from build123d import *

# Parameters (mm, degrees)
SKETCH1_R                = 2.75
BOSS_EXTRUDE1_DEPTH      = 12
BOSS_EXTRUDE2_DEPTH      = 30
BOSS_EXTRUDE2_DEPTH_BACK = 10
CHAMFER1_SIZE            = 17.501152045
CHAMFER1_SIZE_2          = 15
SKETCH4_R                = 2
CUT_EXTRUDE1_DEPTH       = 30
CHAMFER2_SIZE            = 1.5
CUT_EXTRUDE2_DEPTH       = 30
CUT_EXTRUDE2_DEPTH_BACK  = 4
SKETCH5_R                = 5.5
CHAMFER3_SIZE            = 3
BOSS_EXTRUDE3_DEPTH      = 10


with BuildPart() as part:
    # Sketch1 → Boss-Extrude1 (new body)
    with BuildSketch(Plane.XY):
        with BuildLine():
            Line((0, 55), (-15, 55))
            Line((-15, 55), (-10.865898, 24.40520649))
            Line((-10.865898, 24.40520649), (-9.354942791, 21.011545526))
            ThreePointArc((-9.354942791, 21.011545526), (-9.852249787, 20.783002048), (-10.343977944, 20.542690191))
            Line((-10.343977944, 20.542690191), (-7.432453853, -1.004305596))
            ThreePointArc((-7.432453853, -1.004305596), (-4.935468976, -5.647224627), (0, -7.5))
            Line((0, -7.5), (0, -2.75))
            ThreePointArc((0, -2.75), (-2.75, 0), (0, 2.75))
            Line((0, 2.75), (0, 55))
        make_face()
        with Locations((-6.077686218, 34.468271355)):
            Circle(SKETCH1_R, mode=Mode.SUBTRACT)
    extrude(amount=BOSS_EXTRUDE1_DEPTH)

    # Sketch3 → Boss-Extrude2 (add, two sides: drawn at the far end of the back side and taken through both)
    with BuildSketch(Plane(origin=(0, 55, 0), x_dir=(1, 0, 0), z_dir=(0, 1, 0)).offset(-BOSS_EXTRUDE2_DEPTH_BACK)):
        Polygon((0, -17), (-19.25, -17), (-19.25, 10), (-11.25, 10), (-11.25, -12), (0, -12), align=None)
    extrude(amount=BOSS_EXTRUDE2_DEPTH + BOSS_EXTRUDE2_DEPTH_BACK)

    # Chamfer1
    # the kernel refuses this chamfer: 17.501152045, 15 mm, written as the material it adds along each edge
    with BuildSketch(Plane(origin=(-13.648756365, 45, 12), x_dir=(0.1571469904838525, -0.9875752241636421, 0), z_dir=(0, 0, -1))) as chamfer1_piece_1_section:
        Polygon((CHAMFER1_SIZE * 0.999724117502, CHAMFER1_SIZE * 0.0234880574124), (-CHAMFER1_SIZE_2 * 0.157146990484, CHAMFER1_SIZE_2 * 0.987575224164), (0, 0), align=None)
    chamfer1_piece_1 = extrude(amount=12, mode=Mode.PRIVATE)
    chamfer1_piece_1 = split(chamfer1_piece_1, bisect_by=Plane(origin=(-19.25, 37.743808278, 6), z_dir=(1, 0, 0)), keep=Keep.TOP, mode=Mode.PRIVATE)
    add(chamfer1_piece_1)
    # the kernel refuses this chamfer: 17.501152045, 15 mm, written as the material it adds along each edge
    with BuildSketch(Plane(origin=(0, 45, 12), x_dir=(0, 0.02749587661058632, 0.9996219169112968), z_dir=(-1, 0, 0))) as chamfer1_2_piece_1_section:
        Polygon((CHAMFER1_SIZE_2 * 0.999621916911, -CHAMFER1_SIZE_2 * 0.0274958766106), (-CHAMFER1_SIZE_2 * 0.0274958766106, -CHAMFER1_SIZE_2 * 0.999621916911), (0, 0), align=None)
    chamfer1_2_piece_1 = extrude(amount=19.25, mode=Mode.PRIVATE)
    chamfer1_2_piece_1 = chamfer1_2_piece_1 - Plane(origin=(-6.077686218, 34.468271355, 14.181154437), x_dir=(1, 0, 0), z_dir=(0, 0, -1)) * Cylinder(2.75, 99, mode=Mode.PRIVATE)
    chamfer1_2_piece_1 = split(chamfer1_2_piece_1, bisect_by=Plane(origin=(-16.223862411, 32.575106046, 14.181154437), z_dir=(0.7071067811865486, 0.7071067811865466, 0)), keep=Keep.TOP, mode=Mode.PRIVATE)
    chamfer1_2_piece_1 = split(chamfer1_2_piece_1, bisect_by=Plane(origin=(-9.68028065, 39.118687807, 17), z_dir=(0, 0, -1)), keep=Keep.TOP, mode=Mode.PRIVATE)
    add(chamfer1_2_piece_1)

    # Sketch4 → Cut-Extrude1 (cut)
    with BuildSketch(Plane.ZY.offset(19.25)):
        with Locations((1, 70)):
            Circle(SKETCH4_R)
    extrude(amount=-CUT_EXTRUDE1_DEPTH, mode=Mode.SUBTRACT)

    # Chamfer2
    chamfer2_edges = [part.edges().sort_by_distance(p)[0] for p in [
        (-19.25, 70, -1),
    ]]
    chamfer(chamfer2_edges, length=CHAMFER2_SIZE)

    # Sketch5 → Cut-Extrude2 (cut, two sides: drawn at the far end of the back side and taken through both)
    with BuildSketch(Plane.XY.offset(12).offset(-CUT_EXTRUDE2_DEPTH_BACK)):
        Circle(SKETCH5_R)
        with Locations(Location((-6.077686218, 34.468271355, 0), (0, 0, 180))):
            Circle(SKETCH5_R)
    extrude(amount=CUT_EXTRUDE2_DEPTH + CUT_EXTRUDE2_DEPTH_BACK, mode=Mode.SUBTRACT)

    # Chamfer3
    # the kernel refuses this chamfer: 3 mm, written as the material it takes off along each edge
    with BuildSketch(Plane(origin=(0, 0, 8), x_dir=(0.9999950652018582, -0.003141587485879657, 0), z_dir=(0.003141587485879657, 0.9999950652018582, 0))) as chamfer3_piece_1_section:
        Polygon((2.75, CHAMFER3_SIZE), (2.75 + CHAMFER3_SIZE, 0), (2.75, 0), align=None)
    chamfer3_piece_1 = revolve(axis=Axis((0, 0, 8), (0, 0, -1)), revolution_arc=359.64, mode=Mode.PRIVATE)
    chamfer3_piece_1 = chamfer3_piece_1 & Plane(origin=(0, 0, 6.366829543), x_dir=(1, 0, 0), z_dir=(0, 0, 1)) * Cylinder(5.5, 24, mode=Mode.PRIVATE)
    add(chamfer3_piece_1, mode=Mode.SUBTRACT)
    with BuildSketch(Plane(origin=(-6.077686218, 34.468271355, 8), x_dir=(1, 0, 0), z_dir=(0, 1, 0))) as chamfer3_piece_2_section:
        Polygon((2.75, CHAMFER3_SIZE), (2.75 + CHAMFER3_SIZE, 0), (2.75, 0), align=None)
    chamfer3_piece_2 = revolve(axis=Axis((-6.077686218, 34.468271355, 8), (0, 0, -1)), mode=Mode.PRIVATE)
    chamfer3_piece_2 = chamfer3_piece_2 & Plane(origin=(-6.077686218, 34.468271355, 6.366840969), x_dir=(-1, 0, 0), z_dir=(0, 0, 1)) * Cylinder(5.5, 23, mode=Mode.PRIVATE)
    add(chamfer3_piece_2, mode=Mode.SUBTRACT)

    # Sketch6 → Boss-Extrude3 (add)
    with BuildSketch(Plane(origin=(0, 0, 0), x_dir=(-1, 0, 0), z_dir=(0, 0, -1))):
        with BuildLine():
            Line((19.25, 42.201895692), (19.25, 55))
            Line((19.25, 55), (0, 55))
            Line((0, 55), (0, 46.384938288))
            ThreePointArc((0, 46.384938288), (9.849623665, 45.327115656), (19.25, 42.201895692))
        make_face()
    extrude(amount=BOSS_EXTRUDE3_DEPTH)

    # Mirror1: part across plane


with BuildPart() as part_1:
    add(part.part)
    add(part.part.mirror(Plane(origin=(0, 0, 12), x_dir=(0, 0, 1), z_dir=(-1, 0, 0))))


solid = part_1.part
Design review of the part built by this model. Coordinates are the model's own, in mm. A direction names the side the tool comes from. Give positions to 0.01 mm unless a question says otherwise; leave off trailing zeros. Order: outer loops, then holes, each group sorted by start corner. A loop starts at its lowest first (then second) coordinate and runs counter-clockwise, first axis right, second up. Notation, with made-up numbers: (38.25, 61.5) - (55.25, 61.5) arc R22 cw to (55.25, 67.5) - close; hole circle Ø2 at (-10, 4.5). An arc over 180 degrees is marked (long way). Use CSV: the item, a comma, the result in double quotes. Start each with the question number.
Q1. Machinability: for faces 1 (the face through (-11.25, 70, -2)), 2 (the face through (8.91, 9.92, 5.92)), 3 (the face through (4.89, 39.84, 11.28)), 4 (the face through (-10.12, 22.73, 5.92)), 5 (the face through (1, 17, 12)), which of the approach directions +Z, -Z, +X, -X, +Y, -Y give a long, thin tool a straight path to every point of the face, cutting with its end or side? Answer none if there is none.
Q2. Take a section at C-C (y = 0). State the section outline as (x, z) points, and give its area (3 significant figures).
Q3. For P1, Ø6.5, axis at x = -6.08, y = 34.47, coming from the +Z side; P2, Ø12.5, axis at x = 0, y = 0, coming from the -Z side; P3, Ø1.5, axis at x = -1, y = 13.5, coming from the +Z side, all flat-tipped, find the tip position at first contact; note any pin that passes through.
Q4. For line 1 (X direction, y = 67, z = 6); line 2 (Z direction, x = 7, y = 68); line 3 (Z direction, x = -3, y = 9.5), list the stretches that pass through material, from the lowest coordinate up.
Q5. Take a section at B-B (z = 1). Count the separate pieces of the cut face and the enclosed holes in it, and give its area (3 significant figures).
Q6. Take a section at D-D (x = -15). State the section outline as (y, z) points, and give its area (3 significant figures).
Q7. Draft analysis for pull direction Z (two halves, no side actions). For faces 6 (the face through (0, 54, -10)), 7 (the face through (-15, 72, 1)), 8 (the face through (11.09, 26.05, 5.92)), state which applies: pulls with the +Z half, pulls with the -Z half, needs draft (parallel to the pull), parting line crosses it, or undercut.
Q8. Take a section at A-A (y = 70). State the section outline as (x, z) points, and give its area (3 significant figures).
Calculated:
1,face 1,"-Z, +Y"
1,face 2,"+Z, -Z, +X, -Y"
1,face 3,"+Z"
1,face 4,"+Z, -Z, -X"
1,face 5,"+Z, +X, -X, -Y"
2,outline,"(-7.57, 0) - (-2.75, 0) - (-2.75, 5) - (-5.5, 7.75) - (-5.5, 12) - (-7.57, 12) - close; (2.75, 0) - (7.57, 0) - (7.57, 12) - (5.5, 12) - (5.5, 7.75) - (2.75, 5) - close"
2,area,"84.7 mm²"
3,P1,"stops at z = 5.5"
3,P2,"stops at z = 0"
3,P3,"stops at z = 12"
4,line 1,"x = -19.25 to -11.25, 11.25 to 19.25"
4,line 2,"z = 12 to 17"
4,line 3,"z = 0 to 12"
5,separate pieces,"3"
5,enclosed holes,"3"
5,area,"1,940 mm²"
6,outline,"(31.35, 0) - (43.89, 0) - (43.89, -10) - (85, -10) - (85, 17) - (35, 17) - (31.35, 13.35) - close; hole circle Ø4 at (70, 1)"
6,area,"1,300 mm²"
7,face 6,"pulls with the -Z half"
7,face 7,"undercut"
7,face 8,"needs draft"
8,outline,"(-19.25, -10) - (-11.25, -10) - (-11.25, -1) - (-17.75, -1) - (-19.25, -2.5) - close; (-19.25, 4.5) - (-17.75, 3) - (-11.25, 3) - (-11.25, 12) - (11.25, 12) - (11.25, 3) - (17.75, 3) - (19.25, 4.5) - (19.25, 17) - (-19.25, 17) - close; (11.25, -10) - (19.25, -10) - (19.25, -2.5) - (17.75, -1) - (11.25, -1) - close"
8,area,"476 mm²"
